For this review, take the finished solid that the model builds, in its own axes (mm). Face numbers are marked on the shaded views. A direction names the side the tool comes from. Round coordinates to 2 decimals unless told otherwise and drop trailing zeros. Order: outer loops, then holes, each group sorted by start corner. A loop starts at its lowest first (then second) coordinate and runs counter-clockwise, first axis right, second up. Notation, with made-up numbers: M -13.75,-5.75 L 25.25,-5.75 A23 cw 25.25,22.25 Z; hole C 6,-12.5 d7. An arc over 180 degrees is marked long. Use a Markdown table: item, result.
from build123d import *

# Parameters (mm, degrees)
F1_DEPTH = 862
F2_R     = 14
F3_DEPTH = 5
F5_DEPTH = 5


with BuildPart() as f1:
    # F0 (on Front) → F1 (new body)
    with BuildSketch(Plane.XZ):
        Polygon((0, 100), (0, 0), (100, 0), (100, 5), (5, 5), (5, 100), align=None)
    extrude(amount=F1_DEPTH)

    # F2 (on face) → F3 (cut, through all)
    with BuildSketch(Plane.XY.offset(5)):
        with Locations((52.5, -82.4)):
            Circle(F2_R)
        with Locations((52.5, -812)):
            Circle(F2_R)
    extrude(amount=-F3_DEPTH, mode=Mode.SUBTRACT)

    # F4 (on face) → F5 (cut)
    with BuildSketch(Plane.XY.offset(5)):
        Polygon((5, -3.124347), (100, -62.486935), (100, 0), (5, 0), align=None)
    extrude(amount=-F5_DEPTH, mode=Mode.SUBTRACT)


solid = f1.part
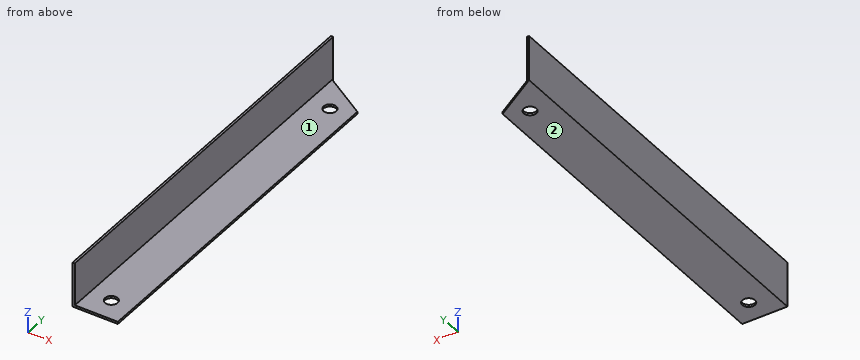
Q1. Wall thickness on line 1 along X through (y, z) = (-812, 1.6); line 2 along Y through (x, z) = (52.5, 1.4); line 3 along Y through (x, z) = (52, 2): over which ranges is each line inside the solid? List them lowest first. Write a range as [from, to].
Determined:
| item | result |
|---|---|
| line 1 | x = [0, 38.5], [66.5, 100] |
| line 2 | y = [-862, -826], [-798, -96.4], [-68.4, -32.81] |
| line 3 | y = [-862, -825.99], [-798.01, -96.39], [-68.41, -32.49] |
Q2. Add section A-A (y = -82.4). Write out the cut boundary in (x, z).
Determined:
| item | result |
|---|---|
| outline | M 0,0 L 38.5,0 L 38.5,5 L 5,5 L 5,100 L 0,100 Z; M 66.5,0 L 100,0 L 100,5 L 66.5,5 Z |
Q3. Add section C-C (z = 46). Write out the cut boundary in (x, y).
Determined:
| item | result |
|---|---|
| outline | M 0,-862 L 5,-862 L 5,0 L 0,0 Z |
Q4. Clearance check with flat-ended pins moving along their axes: pin 1 (10 mm diameter, centred on x = 13, z = 32.5, fed in from +Y); pin 2 (4 mm diameter, centred on x = 69.5, y = -88.5, fed in from -Z); pin 3 (4 mm diameter, centred on y = -301, z = 51, fed in from +X). State where each tip first meets the part, or that it passes through.
Determined:
| item | result |
|---|---|
| pin 1 | passes through |
| pin 2 | stops at z = 0 |
| pin 3 | stops at x = 5 |
Q5. Add section B-B (x = 50). Write out the cut boundary in (y, z).
Determined:
| item | result |
|---|---|
| outline | M -862,0 L -825.77,0 L -825.77,5 L -862,5 Z; M -798.23,0 L -96.17,0 L -96.17,5 L -798.23,5 Z; M -68.63,0 L -31.24,0 L -31.24,5 L -68.63,5 Z |
Q6. Machinability: for the marked faces 1 and 2, which of the approach directions +Z, -Z, +X, -X, +Y, -Y give a long, thin tool a straight path to every point of the face, cutting with its end or side? Answer none if there is none.
Determined:
| item | result |
|---|---|
| face 1 | +Z, +X, +Y, -Y |
| face 2 | -Z, +X, -X, +Y, -Y |
Q7. Add section D-D (y = -180). Write out the cut boundary in (x, z), then the cut area to 3 significant figures.
Determined:
| item | result |
|---|---|
| outline | M 0,0 L 100,0 L 100,5 L 5,5 L 5,100 L 0,100 Z |
| area | 975 mm^2 |
